Autodesk Inventor part; units mm, degrees
ref_plane "YZ Plane" through (0, 0, 0) normal (1, 0, 0) x (0, 1, 0)
ref_plane "XZ Plane" through (0, 0, 0) normal (0, 1, 0) x (-1, 0, 0)
ref_plane "XY Plane" through (0, 0, 0) normal (0, 0, 1) x (1, 0, 0)
sketch "Sketch1" plane through (0, 0, 0) normal (1, 0, 0) x (0, 1, 0)
  line L0 (38.9711, 22.5) -> (38.9711, -22.5)
  line L1 (38.9711, -22.5) -> (0, -45)
  line L2 (0, -45) -> (-38.9711, -22.5)
  line L3 (-38.9711, -22.5) -> (-38.9711, 22.5)
  line L4 (-38.9711, 22.5) -> (0, 45)
  line L5 (0, 45) -> (38.9711, 22.5)
  line L6 (0, 45) -> (0, -45)
  line L7 (38.9711, 0) -> (-38.9711, 0)
  circle A0 centre (38.9711, -22.5) radius 17.5
  circle A1 centre (38.9711, -22.5) radius 12.5
  circle A2 centre (38.9711, -22.5) radius 10.4
  circle A3 centre (38.9711, -22.5) radius 15
  line L8 (38.9711, -22.5) -> (62.5188, -22.5)
  line L9 (53.9711, -26.5) -> (61.9711, -26.5)
  line L10 (61.9711, -26.5) -> (61.9711, -18.5)
  line L11 (61.9711, -18.5) -> (53.9711, -18.5)
  line L12 (53.9711, -18.5) -> (53.9711, -26.5)
  line L13 (53.9711, -26.5) -> (61.9711, -18.5) construction
  line L14 (61.9711, -26.5) -> (53.9711, -18.5) construction
  circle A4 centre (38.9711, 22.5) radius 10.4
  circle A5 centre (38.9711, 22.5) radius 12.5
  circle A6 centre (0, 45) radius 10.4
  circle A7 centre (0, 45) radius 12.5
  circle A8 centre (-38.9711, 22.5) radius 10.4
  circle A9 centre (-38.9711, 22.5) radius 12.5
  circle A10 centre (-38.9711, -22.5) radius 10.4
  circle A11 centre (-38.9711, -22.5) radius 12.5
  circle A12 centre (0, -45) radius 10.4
  circle A13 centre (0, -45) radius 12.5
  line L15 (42.9711, 10.6573) -> (42.9711, -10.6573)
  line L16 (34.9711, 10.6573) -> (34.9711, -10.6573)
  line L17 (12.2561, 42.5427) -> (30.715, 31.8855)
  line L18 (8.2561, 35.6145) -> (26.715, 24.9573)
  line L19 (-30.715, 31.8855) -> (-12.2561, 42.5427)
  line L20 (-26.715, 24.9573) -> (-8.2561, 35.6145)
  line L21 (-42.9711, -10.6573) -> (-42.9711, 10.6573)
  line L22 (-34.9711, -10.6573) -> (-34.9711, 10.6573)
  line L23 (-12.2561, -42.5427) -> (-30.715, -31.8855)
  line L24 (-8.2561, -35.6145) -> (-26.715, -24.9573)
  line L25 (30.715, -31.8855) -> (12.2561, -42.5427)
  line L26 (26.715, -24.9573) -> (8.2561, -35.6145)
  line L27 (38.9711, 22.5) -> (0, 0)
  line L28 (28.9786, 19.6175) -> (27.1145, 18.5413)
  line L29 (31.4786, 15.2874) -> (29.6145, 14.2112)
  line L30 (29.9645, 17.3) -> (28.1458, 16.25)
  arc A14 (31.4786, 15.2874) -> (28.9786, 19.6175) centre (30.2286, 17.4525) ccw
  arc A15 (27.1145, 18.5413) -> (29.6145, 14.2112) centre (28.3645, 16.3763) ccw
  arc A16 (2.5, 34.905) -> (-2.5, 34.905) centre (0, 34.905) ccw
  line L31 (2.5, 34.905) -> (2.5, 32.7526)
  line L32 (-2.5, 34.905) -> (-2.5, 32.7526)
  arc A17 (-2.5, 32.7526) -> (2.5, 32.7526) centre (0, 32.7526) ccw
  arc A18 (-28.9786, 19.6175) -> (-31.4786, 15.2874) centre (-30.2286, 17.4525) ccw
  line L33 (-28.9786, 19.6175) -> (-27.1145, 18.5413)
  line L34 (-31.4786, 15.2874) -> (-29.6145, 14.2112)
  arc A19 (-29.6145, 14.2112) -> (-27.1145, 18.5413) centre (-28.3645, 16.3763) ccw
  arc A20 (-31.4786, -15.2874) -> (-28.9786, -19.6175) centre (-30.2286, -17.4525) ccw
  line L35 (-31.4786, -15.2874) -> (-29.6145, -14.2112)
  line L36 (-28.9786, -19.6175) -> (-27.1145, -18.5413)
  arc A21 (-27.1145, -18.5413) -> (-29.6145, -14.2112) centre (-28.3645, -16.3763) ccw
  arc A22 (-2.5, -34.905) -> (2.5, -34.905) centre (0, -34.905) ccw
  line L37 (-2.5, -34.905) -> (-2.5, -32.7526)
  line L38 (2.5, -34.905) -> (2.5, -32.7526)
  arc A23 (2.5, -32.7526) -> (-2.5, -32.7526) centre (0, -32.7526) ccw
  arc A24 (28.9786, -19.6175) -> (31.4786, -15.2874) centre (30.2286, -17.4525) ccw
  line L39 (28.9786, -19.6175) -> (27.1145, -18.5413)
  line L40 (31.4786, -15.2874) -> (29.6145, -14.2112)
  arc A25 (29.6145, -14.2112) -> (27.1145, -18.5413) centre (28.3645, -16.3763) ccw
  line L41 (-48.9711, -15) -> (-48.9711, 15)
  line L42 (-48.9711, 15) -> (-56.9711, 15)
  line L43 (-56.9711, 15) -> (-56.9711, -15)
  line L44 (-56.9711, -15) -> (-48.9711, -15)
  circle A26 centre (-38.9711, -22.5) radius 17.5
  circle A27 centre (-38.9711, 22.5) radius 17.5
  line L45 (-52.9711, -15) -> (-52.9711, 15)
  circle A28 centre (38.9711, 22.5) radius 2
  circle A29 centre (0, 45) radius 2
  circle A30 centre (-38.9711, 22.5) radius 2
  circle A31 centre (-38.9711, -22.5) radius 2
  circle A32 centre (0, -45) radius 2
  circle A33 centre (38.9711, -22.5) radius 2
  point P0 (57.9711, -22.5)
  point P1 (-42.9711, 10.6573)
  dimension "d0" = 35
  dimension "d1" = 45
  dimension "d2" = 25
  dimension "d3" = 20.8
  dimension "d4" = 30
  dimension "d5" = 8
  dimension "d6" = 8
  dimension "d9" = 360
  dimension "d11" = 4
  dimension "d12" = 4
  dimension "d15" = 360
  dimension "d17" = 2.5
  dimension "d18" = 2.5
  dimension "d22" = 360
  dimension "d24" = 30
  dimension "d25" = 8
  dimension "d26" = 30
  dimension "d28" = 35
  dimension "d29" = 35
  dimension "d30" = 4
  dimension "d35" = 4
  dimension "d38" = 360
extrude "Extrusion1" add sketch "Sketch1" against normal blind 18 contours L5 A28 L0 | L27 A28 L5 | L0 A28 L27 | A28 L5 A4 L0 | L0 A4 A14 L27 A28 | A28 L27 A14 A4 L5 | A4 L5 A5 L0 | L0 A5 L29 A4 | A4 L28 A5 L5 | A14 A4 L27 | L27 A4 A14 | A5 L15 A0 L0 | L0 L7 L16 A5 | L29 A5 L27 A4 | A5 L18 A7 L5 | L5 A7 L17 A5 | A4 L27 A5 L28 | L0 A0 L16 L7 | A7 L31 A6 L5 | L5 A6 L4 A7 | A0 L15 A3 L0 | L0 A3 L16 A0 | A6 A16 L6 A29 L5 | L5 A29 L4 A6 | A3 L15 A1 L0 | L0 A1 L16 A3 | A29 L6 L5 | L5 L4 A29 | L31 A7 L6 A6 | A6 L6 A16 | A1 L8 A2 L0 | L0 A2 L40 A1 | L26 A3 L1 A0 | A0 L1 A13 L26 | L6 A29 L4 | L6 A16 A6 L4 A29 | A6 A16 L6 | L6 A7 L32 A6 | A6 L32 A7 L4 | A7 L4 A27 L19 | A2 L8 A33 L0 | L0 A33 L1 A2 A24 | L26 A1 L1 A3 | A0 L25 A13 L1 | L1 A3 L25 A0 | A13 L1 A12 L38 | A13 L38 A12 L6 | L6 A12 L37 A13 | L37 A12 L2 A13 | A3 L1 A1 L25 | A1 L1 A2 L8 | A7 L20 A27 L4 | A27 L4 A9 L19 | A33 L8 L0 | L0 L1 A33 | A2 L1 A33 L8 | A24 A2 | A2 L39 A1 L40 | A1 L39 A2 L1 | A13 L2 A12 L1 | A12 A22 L6 | L6 A22 A12 | A12 L1 A32 L6 A22 | A13 L2 A26 L24 | A22 L6 A32 L2 A12 | A11 L35 A10 L3 | A9 L3 A8 L34 | A27 L20 A9 L4 | A9 L4 A8 L3 | A27 L45 A26 L44 L43 L42 | L42 L45 A27 | L8 A33 L1 | A12 L2 A32 L1 | A13 L23 A26 L2 | A26 L2 A11 L24 | L3 A10 L2 A11 | A26 L41 A27 L21 | L21 A11 L41 A26 | A27 L41 A9 L21 | A11 L36 A10 L35 | L34 A8 L33 A9 | A9 L33 A8 L4 | L41 A27 L45 L42 | A27 L41 A26 L45 | A32 L2 L1 | L1 L6 A32 | L6 L2 A32 | A26 L23 A11 L2 | A11 L2 A10 L36 | A10 A20 L2 A31 L3 | L3 A31 L2 A10 | L41 L44 L45 A26 | A8 L4 A30 L3 | L3 A30 L4 A8 A18 | A10 A20 | A18 A8 | L45 L44 A26 | A31 L2 L3 | L3 L2 A31 | A30 L4 L3 | L3 L4 A30
extrude "Extrusion2" cut sketch "Sketch1" against normal blind 15 contours L5 A28 L0 | L27 A28 L5 | L0 A28 L27 | A28 L5 A4 L0 | L0 A4 A14 L27 A28 | A28 L27 A14 A4 L5 | A14 A4 L27 | L27 A4 A14 | A6 A16 L6 A29 L5 | L5 A29 L4 A6 | A29 L6 L5 | L5 L4 A29 | A6 L6 A16 | L6 A29 L4 | L6 A16 A6 L4 A29 | A6 A16 L6 | A2 L8 A33 L0 | L0 A33 L1 A2 A24 | A33 L8 L0 | L0 L1 A33 | A2 L1 A33 L8 | A24 A2 | A12 A22 L6 | L6 A22 A12 | A12 L1 A32 L6 A22 | A22 L6 A32 L2 A12 | L8 A33 L1 | A12 L2 A32 L1 | A32 L2 L1 | L1 L6 A32 | L6 L2 A32 | A10 A20 L2 A31 L3 | L3 A31 L2 A10 | A8 L4 A30 L3 | L3 A30 L4 A8 A18 | A10 A20 | A18 A8 | A31 L2 L3 | L3 L2 A31 | A30 L4 L3 | L3 L4 A30
extrude "Extrusion3" cut sketch "Sketch1" against normal blind 18 contours L5 A28 L0 | L27 A28 L5 | L0 A28 L27 | A14 A4 L27 | L27 A4 A14 | L29 A5 L27 A4 | A4 L27 A5 L28 | A29 L6 L5 | L5 L4 A29 | L31 A7 L6 A6 | A6 L6 A16 | L6 A29 L4 | A6 A16 L6 | L6 A7 L32 A6 | A13 L38 A12 L6 | L6 A12 L37 A13 | A33 L8 L0 | L0 L1 A33 | A24 A2 | A2 L39 A1 L40 | A12 A22 L6 | L6 A22 A12 | L8 A33 L1 | A11 L36 A10 L35 | L34 A8 L33 A9 | A32 L2 L1 | L1 L6 A32 | L6 L2 A32 | A10 A20 | A18 A8 | A31 L2 L3 | L3 L2 A31 | A30 L4 L3 | L3 L4 A30
extrude "Extrusion4" add sketch "Sketch1" against normal blind 32 contours A27 L45 A26 L44 L43 L42 | L42 L45 A27 | L45 L44 A26
sketch "Sketch2" plane through (0, 0, 0) normal (0, 0, 1) x (1, 0, 0)
  line L0 (-18, -42.9711) -> (-32, -52.9711)
  line L1 (-18, -30.715) -> (-18, -51.4711)
  line L2 (-18, -46.6579) -> (-26.8386, -52.9711)
  line L3 (-18, -52.9711) -> (-32, -52.9711)
  point P0 (0, 0)
  point P1 (-18, -48.9711)
  point P2 (-22.4193, -49.8145)
  dimension "d44" = 3
extrude "Extrusion5" add sketch "Sketch2" along normal mid plane 5
sketch "Sketch3" plane through (0, -56.9711, -15) normal (0, -1, 0) x (1, 0, 0)
  line L0 (0, 30) -> (0, 0)
  line L1 (0, 30) -> (-32, 30)
  line L2 (-32, 0) -> (-32, 30)
  line L3 (0, 0) -> (-32, 0)
  line L4 (-32, 0) -> (0, 30)
  line L5 (-6, 25) -> (-26, 25)
  line L6 (-26, 25) -> (-26, 5)
  line L7 (-26, 5) -> (-6, 5)
  line L8 (-6, 5) -> (-6, 25)
  line L9 (-6, 25) -> (-26, 5) construction
  line L10 (-26, 25) -> (-6, 5) construction
  circle A0 centre (-26, 25) radius 1.5
  circle A1 centre (-26, 5) radius 1.5
  circle A2 centre (-6, 5) radius 1.5
  circle A3 centre (-6, 25) radius 1.5
  point P0 (0, 15)
  point P1 (-16, 15)
  dimension "d47" = 20
  dimension "d48" = 20
  dimension "d49" = 3
  dimension "d52" = 360
extrude "Extrusion6" cut sketch "Sketch3" against normal blind 5 contours A1 L6 L4 | L4 L6 L7 A1 | A0 L6 L5 | L5 L6 A0 | L6 A1 L4 | L4 A1 L7 L6
equation "\"d6\" = d5"
equation "\"d12\" = d11"
equation "\"d18\" = d17"
properties part number "support_electrical_magnets"
Geometry: final body of the model. Coordinates: model frame, mm. A direction names the side the tool comes from. Give positions to 0.01 mm unless a question says otherwise; leave off trailing zeros. Write each loop counter-clockwise with the first axis right and the second up, starting at its lowest first coordinate (ties: lowest second). Pieces come first, ordered by that corner, then holes. Notation, with made-up numbers: (66, -23) - (86, -23) arc R28 cw to (86, 15) - close; hole circle Ø8 at (-20, 67.5). An arc over 180 degrees is marked (long way). Return JSON: item names as keys, results as strings. Group by question number.
1) Section B-B on x = -29. Return the cut outline in (y, z), plus the area to 3 significant figures.
2) First-contact query: P1, Ø2.5, axis at x = -7, z = 33.5, coming from the +Y side; P2, Ø3, axis at x = -25.5, y = -46, coming from the +Z side; P3, Ø5, axis at x = -26, z = 10, coming from the +Y side; P4, Ø3, axis at x = -3.5, y = 24, coming from the -Z side. Flat tips, straight axial feed; report the tip coordinate or a pass-through.
3) Set-up query: faces 1 (the flat face through (-15, 41.14, 22.65)), 2 (the flat face through (-8.87, 17.36, 30.36)), 3 (the flat face through (-24, -49, 2.5)). Return all of +Z, -Z, +X, -X, +Y, -Y with unobstructed straight access to the full face (end or side cutting, diameter ignored); none if empty.
4) Mould query, pull axis Z, two halves, no side actions, for faces 4 (the cylindrical face through (-8.87, 26.5, -21.68)), 5 (the flat face through (-24.9, -47.9, 0)), 6 (the flat face through (-24, -49, -2.5)), 7 (the flat face through (-15, 41.14, -22.35)). Classes: released by +Z, released by -Z, zero draft, split by the parting line, or undercut.
5) Section A-A on y = 0. Return the cut outline in (x, z) (3 decimals).
6) Section C-C on z = 49. Return the cut outline in (x, y), plus the area to 3 significant figures.
7) Line query: line 1 (Y direction, x = -6.75, z = -22.5); line 2 (Z direction, x = -14, y = 38); line 3 (Y direction, x = -1.5, z = 21.5). Output: solid intervals per line, ascending.
Filled in:
{
 "1": {"outline": "(-56.97, -15) - (-52.97, -15) - (-52.97, -2.5) - (-50.83, -2.5) - (-50.83, 2.5) - (-52.97, 2.5) - (-52.97, 15) - (-56.97, 15) - close", "area": "131 mm^2"},
 "2": {"P1": "stops at y = 46.79", "P2": "passes through", "P3": "stops at y = -52.97", "P4": "stops at z = -36.63"},
 "3": {"face 1": "+X", "face 2": "+X, -X", "face 3": "+Z, -X, +Y"},
 "4": {"face 4": "undercut", "face 5": "zero draft", "face 6": "released by -Z", "face 7": "undercut"},
 "5": {"outline": "(-18, -57.5) - (0, -57.5) - (0, -55.4) - (-15, -55.4) - (-15, -47) - (-18, -47) - close; (-18, -43) - (-15, -43) - (-15, -37.405) - (-18, -37.405) - close; (-18, 37.405) - (-15, 37.405) - (-15, 43) - (-18, 43) - close; (-18, 47) - (-15, 47) - (-15, 55.4) - (0, 55.4) - (0, 57.5) - (-18, 57.5) - close"},
 "6": {"outline": "(-18, -11.84) - (0, -11.84) - (0, -9.6) - (-15, -9.6) - (-15, 9.6) - (0, 9.6) - (0, 11.84) - (-18, 11.84) - close", "area": "138 mm^2"},
 "7": {"line 1": "y = -51.47 to -49.37, -28.57 to -26.47, 26.47 to 28.57, 49.37 to 51.47", "line 2": "z = -34.96 to -32.85, -12.15 to 12.15, 32.85 to 34.96", "line 3": "y = -51.43 to -49.32, -28.62 to -26.51, 26.51 to 28.62, 49.32 to 51.43"}
}
